Input: part model. Units: mm. Frame: model coordinates. Give positions to 0.01 mm unless a question says otherwise; leave off trailing zeros. Loops run counter-clockwise (first coordinate to the right, second up) from the corner with the lowest first, then second, coordinate; pieces in that order, holes last. Notation, with made-up numbers: M -39,-14 L 11,-14 A33 cw 11,16 Z; hole C 80.5,80 d2. An arc over 180 degrees is marked long. One line per item, written item: value. Start each with the question number.
(1) Section A-A on x = 2.5. Output: boundary loops of the cut face in (y, z).
(2) Pull-direction query (Y, two-part tool) for faces 1 (the conical face through (0.13, -3.12, -5.38)), 2 (the conical face through (6.27, 3.12, -5.38)), 3 (the cylindrical face through (3.245, -3.905, 0.867)); classes: released by +Y, released by -Y, zero draft, split by the parting line, or undercut.
(3) Pin query (flat end, axial travel): P1, Ø3, axis at x = 2, z = 2.5, coming from the +Y side. Return the tip coordinate at first contact, or that it passes through.
(4) Ray query, line 1 along Z through (x, y) = (5, 1.75); line 2 along Z through (x, y) = (4.5, -1); line 3 along Y through (x, z) = (2, 3). Return the intervals inside material, ascending. Write a range as from..to.
```python
from build123d import *

# Parameters (mm, degrees)
CROQUIS1_W            = 6.4
CROQUIS1_H            = 6.92
CORTAR_EXTRUIR1_DEPTH = 7
CROQUIS3_OUTSIDE_W    = 42.114
CROQUIS3_OUTSIDE_H    = 43.968
CROQUIS3_OUTSIDE_R    = 5.992895794
CORTAR_EXTRUIR2_DEPTH = 7
CORTAR_EXTRUIR2_TAPER = 60
CROQUIS5_OUTSIDE_W    = 21.33
CROQUIS5_OUTSIDE_H    = 23.184
CROQUIS5_OUTSIDE_R    = 5.992895794
CORTAR_EXTRUIR3_DEPTH = 1
CORTAR_EXTRUIR3_TAPER = 60
CROQUIS6_R            = 4
CORTAR_EXTRUIR4_DEPTH = 7


with BuildPart() as part:
    # Croquis1 → Revolución1 (revolve)
    with BuildSketch(Plane.XY):
        with Locations((3.2, 3.46)):
            Rectangle(CROQUIS1_W, CROQUIS1_H)
    revolve(axis=Axis((6.4, 0, 0), (-1, 0, 0)))

    # Croquis2 → Cortar-Extruir1 (cut)
    with BuildSketch(Plane(origin=(6.4, 0, 0), x_dir=(0, 0, -1), z_dir=(1, 0, 0))):
        with BuildLine():
            Line((-5.992895794, -3.46), (-5.992895794, 3.46))
            ThreePointArc((-5.992895794, 3.46), (-6.92, 0), (-5.992895794, -3.46))
        make_face()
        with BuildLine():
            Line((-5.992895794, 3.46), (0, 6.92))
            ThreePointArc((0, 6.92), (-3.46, 5.992895794), (-5.992895794, 3.46))
        make_face()
        with BuildLine():
            ThreePointArc((5.992895794, 3.46), (3.46, 5.992895794), (0, 6.92))
            Line((0, 6.92), (5.992895794, 3.46))
        make_face()
        with BuildLine():
            ThreePointArc((6.92, 0), (6.684206718, 1.791027792), (5.992895794, 3.46))
            Line((5.992895794, 3.46), (5.992895794, -3.46))
            ThreePointArc((5.992895794, -3.46), (6.684206718, -1.791027792), (6.92, 0))
        make_face()
        with BuildLine():
            ThreePointArc((0, -6.92), (3.46, -5.992895794), (5.992895794, -3.46))
            Line((5.992895794, -3.46), (0, -6.92))
        make_face()
        with BuildLine():
            Line((0, -6.92), (-5.992895794, -3.46))
            ThreePointArc((-5.992895794, -3.46), (-3.46, -5.992895794), (0, -6.92))
        make_face()
    extrude(amount=-CORTAR_EXTRUIR1_DEPTH, mode=Mode.SUBTRACT)

    # Croquis3 outside → Cortar-Extruir2 (cut)
    with BuildSketch(Plane(origin=(6.4, 0, 0), x_dir=(0, 0, -1), z_dir=(1, 0, 0))):
        Rectangle(CROQUIS3_OUTSIDE_W, CROQUIS3_OUTSIDE_H)
        Circle(CROQUIS3_OUTSIDE_R, mode=Mode.SUBTRACT)
    extrude(amount=-CORTAR_EXTRUIR2_DEPTH, taper=CORTAR_EXTRUIR2_TAPER, mode=Mode.SUBTRACT)

    # Croquis5 outside → Cortar-Extruir3 (cut)
    with BuildSketch(Plane.ZY):
        Rectangle(CROQUIS5_OUTSIDE_W, CROQUIS5_OUTSIDE_H)
        Circle(CROQUIS5_OUTSIDE_R, mode=Mode.SUBTRACT)
    extrude(amount=-CORTAR_EXTRUIR3_DEPTH, taper=CORTAR_EXTRUIR3_TAPER, mode=Mode.SUBTRACT)

    # Croquis6 → Cortar-Extruir4 (cut)
    with BuildSketch(Plane(origin=(6.4, 0, 0), x_dir=(0, 0, -1), z_dir=(1, 0, 0))):
        Circle(CROQUIS6_R)
    extrude(amount=-CORTAR_EXTRUIR4_DEPTH, mode=Mode.SUBTRACT)


solid = part.part
```
Output values:
1. outline: M -6.92,0 L -3.46,-5.99 L 3.46,-5.99 L 6.92,0 L 3.46,5.99 L -3.46,5.99 Z; hole C 0,0 d8
2. face 1: released by -Y
2. face 2: released by +Y
2. face 3: undercut
3. P1: stops at y = 6.34
4. line 1: z = -5.99..-3.6, 3.6..5.99
4. line 2: z = -5.99..-3.87, 3.87..5.99
4. line 3: y = -5.19..-2.65, 2.65..5.19
